Check sheet for the modelled part. Datum: model origin and axes. Units: mm. Give positions to 0.01 mm unless a question says otherwise; leave off trailing zeros. Order: outer loops, then holes, each group sorted by start corner. A loop starts at its lowest first (then second) coordinate and runs counter-clockwise, first axis right, second up. Notation, with made-up numbers: (34, 34.25) -> (58, 34.25) arc R35 cw to (58, 73.25) -> close; hole circle Ø10 at (56, 42.25). An arc over 180 degrees is marked (long way). Write each question's results on one line, items separated by ' | '.
Autodesk Inventor part; units mm, degrees
ref_plane "YZ Plane" through (0, 0, 0) normal (1, 0, 0) x (0, 1, 0)
ref_plane "XZ Plane" through (0, 0, 0) normal (0, 1, 0) x (-1, 0, 0)
ref_plane "XY Plane" through (0, 0, 0) normal (0, 0, 1) x (1, 0, 0)
sketch "Sketch1" plane through (0, 0, 0) normal (0, 0, 1) x (1, 0, 0)
  circle A0 centre (0, 0) radius 2
  line L0 (0, 4.0415) -> (3.5, 2.0207)
  line L1 (3.5, 2.0207) -> (3.5, -2.0207)
  line L2 (3.5, -2.0207) -> (0, -4.0415)
  line L3 (0, -4.0415) -> (-3.5, -2.0207)
  line L4 (-3.5, -2.0207) -> (-3.5, 2.0207)
  line L5 (-3.5, 2.0207) -> (0, 4.0415)
  dimension "Sw" = 7
  dimension "Diameter" = 4
extrude "Extrusion1" add sketch "Sketch1" along normal mid plane 2.9
thread "Thread1"
sketch "Sketch4" plane through (0, 0, 0) normal (0, 1, 0) x (-1, 0, 0)
  line L0 (0, -1.45) -> (0, 1.45)
  line L1 (0, -1.45) -> (-3.5, -1.45)
  line L2 (-3.5, -1.45) -> (-4.0415, -1.1374)
  line L3 (-4.0415, -1.1374) -> (-4.0415, -1.45)
  line L4 (-4.0415, -1.45) -> (-3.5, -1.45)
  line L5 (0, -2.03) -> (0, 2.03)
  dimension "d6" = 4.0415
  dimension "d7" = 30
  dimension "d8" = 3.5
revolve "Revolution1" cut sketch "Sketch4" angle 360 about axis through (0, 0, -10) along (0, 0, 1)
mirror "Mirror1" about plane through (0, 0, 0) normal (0, 0, 1) of "Revolution1"
sketch "Sketch6" plane through (0, 0, -1.45) normal (0, 0, -1) x (-1, 0, 0)
  circle A0 centre (0, 0) radius 2
  circle A1 centre (0, 0) radius 3.8717
  dimension "d15" = 7.7434
extrude "Extrusion3" cut sketch "Sketch6" against normal through all keep common part
chamfer "Chamfer2" distance 0.35 angle 45 1 edges at (-2, 0, -1.45)
sketch "Sketch8" plane through (0, 0, 1.45) normal (0, 0, 1) x (1, 0, 0)
  line L0 (-2.5, 0) -> (3.5, 0)
  circle A0 centre (0, 0) radius 3.15
  circle A1 centre (0, 0) radius 2.1
  dimension "d22" = 6.3
  dimension "d34" = 4.2
extrude "Extrusion6" add sketch "Sketch8" along normal blind 1.995
sketch "Sketch11" plane through (0, 0, 0) normal (0, 1, 0) x (-1, 0, 0)
  line L0 (1.75, -1.45) -> (3.5, -1.45)
  line L1 (3.15, 3.55) -> (0, 3.55)
  line L2 (3.5, 1.45) -> (1.75, 1.45)
  line L3 (3.43, 3.27) -> (3.43, 1.45)
  line L4 (3.15, 1.45) -> (3.15, 3.445)
  line L5 (2.1, 1.45) -> (2.1, 3.445)
  line L6 (0, -2.4616) -> (0, 4.6196)
  arc A0 (3.43, 3.27) -> (3.15, 3.55) centre (3.15, 3.27) ccw
  line L7 (3.15, 3.445) -> (3.038, 3.445)
  line L8 (3.038, 3.445) -> (3.038, 3.55)
  dimension "d35" = 5
  dimension "d36" = 3.43
  dimension "d37" = 0.28
  dimension "d38" = 0.28
  dimension "d40" = 0.392
revolve "Revolution2" add sketch "Sketch11" angle 360 about axis through (0, 0, -10) along (0, 0, 1)
equation "\"d4\" = M"
equation "\"d6\" = 0.57735 * Sw"
equation "\"d8\" = 0.5 * Sw"
equation "\"d15\" = 1.10619 * Sw"
equation "\"d20\" = 0.5 * Pitch"
equation "\"d21\" = 0.5 * Pitch"
equation "\"d22\" = 0.9 * Sw"
equation "\"d34\" = 1.05 * Diameter"
equation "\"d25\" = -0.95 * M + 0.95 * h"
equation "\"d35\" = h"
equation "\"d36\" = 0.49 * Sw"
equation "\"d38\" = d37"
equation "\"d40\" = 1.4 * d38"
properties part number "11-4503" material "Steel, Mild"
1. Section check B-B on z = 0.1. Record the cut outline in (x, y), then the cut area to 3 significant figures.
Verdict:
outline: (-3.5, -1.66) arc R3.87 ccw to (-3.18, -2.2) -> (-0.32, -3.86) arc R3.87 ccw to (0.32, -3.86) -> (3.18, -2.2) arc R3.87 ccw to (3.5, -1.66) -> (3.5, 1.66) arc R3.87 ccw to (3.18, 2.2) -> (0.32, 3.86) arc R3.87 ccw to (-0.32, 3.86) -> (-3.18, 2.2) arc R3.87 ccw to (-3.5, 1.66) -> close; hole circle Ø4 at (0, 0) | area: 29.6 mm^2
2. Section check C-C on z = 1.65. Record the cut outline in (x, y), then the cut area to 3 significant figures.
Verdict:
outline: circle Ø6.86 at (0, 0); hole circle Ø4.2 at (0, 0) | area: 23.1 mm^2
3. Mould release check, pull along X, two halves, no side actions. Record for faces 1 (the cylindrical face through (0, 2, 0)), 2 (the cylindrical face through (2.003, -0.631, 2.434)), 3 (the flat face through (-3.5, 0, 0)), 4 (the cylindrical face through (-3.27, 1.03, 2.35)): +X half, -X half, draft (parallel to the pull), parting line (faces both ways), or undercut.
Verdict:
face 1: undercut | face 2: undercut | face 3: -X half | face 4: parting line
4. Section check A-A on x = 0. Record the cut outline in (y, z) (3 decimals), then the cut area to 3 significant figures.
Verdict:
outline: (-3.872, -1.235) -> (-3.5, -1.45) -> (-2.35, -1.45) -> (-2, -1.1) -> (-2, 1.45) -> (-2.1, 1.45) -> (-2.1, 3.445) -> (-3.038, 3.445) -> (-3.038, 3.55) -> (-3.15, 3.55) arc R0.28 ccw to (-3.43, 3.27) -> (-3.43, 1.45) -> (-3.5, 1.45) -> (-3.872, 1.235) -> close; (2, -1.1) -> (2.35, -1.45) -> (3.5, -1.45) -> (3.872, -1.235) -> (3.872, 1.235) -> (3.5, 1.45) -> (3.43, 1.45) -> (3.43, 3.27) arc R0.28 ccw to (3.15, 3.55) -> (3.038, 3.55) -> (3.038, 3.445) -> (2.1, 3.445) -> (2.1, 1.45) -> (2, 1.45) -> close | area: 15.9 mm^2
5. Gauge pin test, flat ends, axial feed: pin 1 Ø1.5 at (x, z) = (2, -0.5) entering from -Y; pin 2 Ø3 at (x, y) = (0, 0) entering from -Z. Record the tip position at first contact, or that the pin passes through.
Verdict:
pin 1: stops at y = -3.32 | pin 2: passes through
6. Material ranges on probe 1 along X at (y, z) = (0, 0.6); probe 2 along Y at (x, z) = (0, 3.05), recorded low to high. Write a range as from..to.
Verdict:
probe 1: x = -3.5..-2, 2..3.5 | probe 2: y = -3.43..-2.1, 2.1..3.43
